Autodesk Inventor part; units mm, degrees
ref_plane "YZ Plane" through (0, 0, 0) normal (1, 0, 0) x (0, 1, 0)
ref_plane "XZ Plane" through (0, 0, 0) normal (0, 1, 0) x (-1, 0, 0)
ref_plane "XY Plane" through (0, 0, 0) normal (0, 0, 1) x (1, 0, 0)
sketch "Sketch1" plane through (0, 0, 0) normal (0, 1, 0) x (-1, 0, 0)
  line L0 (-3, 0) -> (-13, -10)
  line L1 (-13, -10) -> (-28, -10)
  line L2 (-28, -14) -> (-11.3431, -14)
  line L3 (-11.3431, -14) -> (0, -2.6569)
  line L4 (-28, -10) -> (-28, -14)
  line L5 (-3, 0) -> (0, 0)
  line L6 (0, 0) -> (0, -2.6569)
  dimension "d7" = 15
  dimension "d9" = 4
  dimension "d38" = 10
  dimension "d39" = 4
extrude "Extrusion1" add sketch "Sketch1" along normal blind 20
sketch "Sketch4" plane through (13, 0, -10) normal (0, 0, 1) x (1, 0, 0)
  line L0 (0, 20) -> (15, 20)
  line L1 (15, 0) -> (15, 20)
  point P0 (-13, 0)
  point P1 (10, 15)
  point P2 (10, 5)
  dimension "d28" = 5
  dimension "d29" = 10
  dimension "d40" = 5
hole "Hole3" at (23, 15, -10) at (23, 5, -10) direction (0, 0, -1) diameter 4.5 end through all
fillet "Fillet4" radius 5 5 edges at (28, 20, -12) (28, 0, -12) (11.3431, 10, -14) (13, 10, -10) (3, 10, 0)
mirror "Mirror3" about plane through (0, 0, -2.6569) normal (-1, 0, 0) of "Extrusion1", "Fillet4", "Hole3"
fillet "Fillet5" radius 5 1 edges at (0, 10, -2.6569)
properties part number "clip_cover"
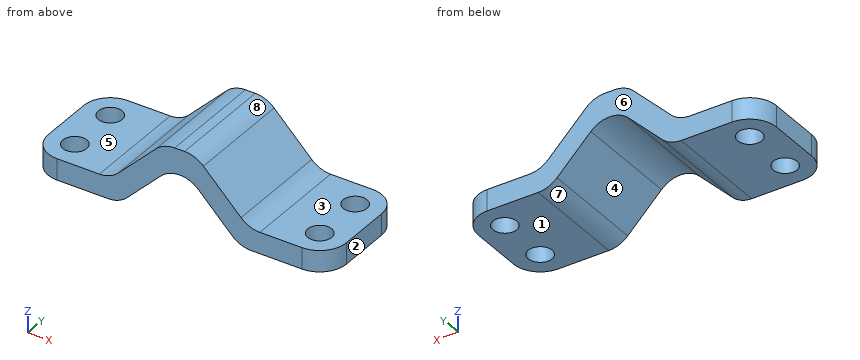
For this review, take the finished solid that the model builds, in its own axes (mm). Face numbers are marked on the shaded views. A direction names the side the tool comes from. Round coordinates to 2 decimals unless told otherwise and drop trailing zeros. Order: outer loops, then holes, each group sorted by start corner. A loop starts at its lowest first (then second) coordinate and runs counter-clockwise, first axis right, second up. Notation, with made-up numbers: M -27,66 L 27,66 A12 cw 27,75 Z; hole C 20,84.5 d1. An arc over 180 degrees is marked long. Use a Markdown table: item, result. Add a question column.
Item 1: Mouldability with a two-part tool opening along X and no side actions: class the marked faces 6, 7 and 8 as released by +X, released by -X, zero draft, split by the parting line, or undercut.
Item 2: Add section A-A, the plane z = -5.5. Give the boundary of the cut face in (x, y).
Item 3: Add section D-D, the plane x = 2.5. Give the boundary of the cut face in (y, z).
Item 4: To check wall thickness, follow line 1 along Y through (x, z) = (-23, -11.75); line 2 along X through (y, z) = (15, -11.8); line 3 along X through (y, z) = (5, -12.8). State the ranges of each line that lie inside material, in increasing order.
Item 5: Tool access review of the marked faces 1, 2, 3, 4 and 5: name each direction out of +Z, -Z, +X, -X, +Y, -Y from which nothing blocks a thin tool from reaching the whole face with its end or side.
Item 6: Insertion check: pin 1 (2 mm diameter, centred on y = 2.5, z = -4.5, fed in from +X); pin 2 (6 mm diameter, centred on x = 23, y = 5, fed in from +Z); pin 3 (1.5 mm diameter, centred on x = 3.5, y = 14, fed in from -Z). Each pin has a flat end and moves straight along its axis. Give the tip position at first contact, or say it passes through.
Item 7: Add section B-B, the plane y = 11. Give the boundary of the cut face in (x, z), then the cut area to 3 significant figures.
Item 8: Add section C-C, the plane x = -18. Give the boundary of the cut face in (y, z), then the cut area to 3 significant figures.
Geometry results:
| question | item | result |
|---|---|---|
| 1 | face 6 | zero draft |
| 1 | face 7 | undercut |
| 1 | face 8 | released by +X |
| 2 | outline | M -8.5,0 L -2.67,0 L -2.67,20 L -8.5,20 Z; M 2.67,0 L 8.5,0 L 8.5,20 L 2.67,20 Z |
| 3 | outline | M 0,-5.4 L 20,-5.4 L 20,-0.25 L 0,-0.25 Z |
| 4 | line 1 | y = 0 to 2.75, 7.25 to 12.75, 17.25 to 20 |
| 4 | line 2 | x = -28 to -25.25, -20.75 to -9.14, 9.14 to 20.75, 25.25 to 28 |
| 4 | line 3 | x = -28 to -25.25, -20.75 to -10.16, 10.16 to 20.75, 25.25 to 28 |
| 5 | face 1 | -Z, +X, -X, +Y, -Y |
| 5 | face 2 | +Z, -Z, +X, +Y, -Y |
| 5 | face 3 | +Z, +X, +Y, -Y |
| 5 | face 4 | -Z, +Y, -Y |
| 5 | face 5 | +Z, -X, +Y, -Y |
| 6 | pin 1 | stops at x = 8.5 |
| 6 | pin 2 | stops at z = -10 |
| 6 | pin 3 | stops at z = -6.91 |
| 7 | outline | M -28,-14 L -13.41,-14 A5 ccw -9.88,-12.54 L -3.54,-6.19 A5 cw 3.54,-6.19 L 9.88,-12.54 A5 ccw 13.41,-14 L 28,-14 L 28,-10 L 15.07,-10 A5 cw 11.54,-8.54 L 4.46,-1.46 A5 ccw 0.93,0 L -0.93,0 A5 ccw -4.46,-1.46 L -11.54,-8.54 A5 cw -15.07,-10 L -28,-10 Z |
| 7 | area | 260 mm² |
| 8 | outline | M 0,-14 L 20,-14 L 20,-10 L 0,-10 Z |
| 8 | area | 80.0 mm² |
